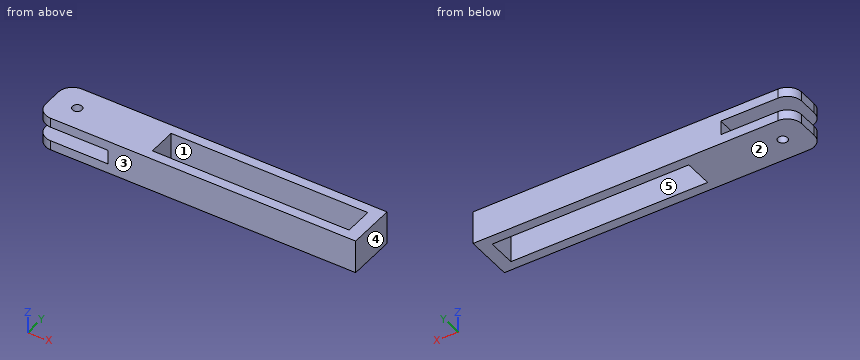
from build123d import *

# Parameters (mm, degrees)
SKETCH3_W           = 206.383928572
SKETCH3_H           = 30
BOSS_EXTRUDE1_DEPTH = 35
CUT_EXTRUDE2_REACH  = 180.273
SKETCH5_W           = 75
SKETCH5_H           = 15
SKETCH6_R           = 5
CUT_EXTRUDE3_DEPTH  = 173.934236055


with BuildPart() as part:
    # Sketch3 → Boss-Extrude1 (new body)
    with BuildSketch(Plane.XY):
        with BuildLine():
            Line((-167.5, 10), (-167.5, -10))
            ThreePointArc((-167.5, -10), (-163.106601718, -20.606601718), (-152.5, -25))
            Line((-152.5, -25), (167.5, -25))
            Line((167.5, -25), (167.5, 25))
            Line((167.5, 25), (-152.5, 25))
            ThreePointArc((-152.5, 25), (-163.106601718, 20.606601718), (-167.5, 10))
        make_face()
        with Locations((50.825520553, 0)):
            Rectangle(SKETCH3_W, SKETCH3_H, mode=Mode.SUBTRACT)
    extrude(amount=BOSS_EXTRUDE1_DEPTH)

    # Sketch5 → Cut-Extrude2 (cut, up to next)
    with BuildSketch(Plane.XZ.offset(25), mode=Mode.PRIVATE) as cut_extrude2_sk1:
        with Locations((-130, 17.5)):
            Rectangle(SKETCH5_W, SKETCH5_H)
    cut_extrude2_tool1 = extrude(cut_extrude2_sk1.sketch, amount=-CUT_EXTRUDE2_REACH, mode=Mode.PRIVATE) & part.part
    add(cut_extrude2_tool1.solids().sort_by_distance((-130, -25, 17.5))[0], mode=Mode.SUBTRACT)

    # Sketch6 → Cut-Extrude3 (cut, through all)
    with BuildSketch(Plane(origin=(0, 0, 0), x_dir=(-1, 0, 0), z_dir=(0, 0, -1))):
        with Locations((141.050190179, 0)):
            Circle(SKETCH6_R)
    extrude(amount=-CUT_EXTRUDE3_DEPTH, mode=Mode.SUBTRACT)


solid = part.part
Input: part model. Units: mm. Frame: model coordinates. Face numbers are marked on the shaded views. A direction names the side the tool comes from. Round coordinates to 2 decimals unless told otherwise and drop trailing zeros. Loops run counter-clockwise (first coordinate to the right, second up) from the corner with the lowest first, then second, coordinate; pieces in that order, holes last. Notation, with made-up numbers: (72.5, -40) -> (84.5, -40) arc R13 ccw to (84.5, -17) -> close; hole circle Ø9 at (25, -1.5). An arc over 180 degrees is marked (long way). Answer as a JSON object with one key per item and string values. Group by question number.
1) Section query C-C on x = 133.5. Output: boundary loops of the cut face in (y, z), plus the area to 3 significant figures.
2) Section query D-D on y = -22. Output: boundary loops of the cut face in (x, z).
3) Section query B-B on y = 0. Output: boundary loops of the cut face in (x, z), plus the area to 3 significant figures.
4) Draft query along X for the marked faces 3, 4 and 5. Return one class per face: +X half, -X half, draft (parallel to the pull), parting line (faces both ways), or undercut.
5) Section query A-A on z = 22. Output: boundary loops of the cut face in (x, y), plus the area to 3 significant figures.
6) Ray query, L1, parallel to Z at x = -145, y = -13; L2, parallel to X at y = -7.5, z = 13.5; L3, parallel to Y at x = 114, z = 4. Return the intervals inside material, ascending.
7) Reachability of the marked faces 1 and 2 from +Z, -Z, +X, -X, +Y, -Y: full face, straight path, thin tool, end or side. Return the list, or none.
8) Pin query (flat end, axial travel): pin 1 (1.5 mm diameter, centred on y = 1, z = 13, fed in from -X); pin 2 (9 mm diameter, centred on x = -141.05, y = 0, fed in from -Z). Return the tip coordinate at first contact, or that it passes through.
Reply:
{
 "1": {"outline": "(-25, 0) -> (-15, 0) -> (-15, 35) -> (-25, 35) -> close; (15, 0) -> (25, 0) -> (25, 35) -> (15, 35) -> close", "area": "700 mm2"},
 "2": {"outline": "(-161.5, 0) -> (167.5, 0) -> (167.5, 35) -> (-161.5, 35) -> (-161.5, 25) -> (-92.5, 25) -> (-92.5, 10) -> (-161.5, 10) -> close"},
 "3": {"outline": "(-167.5, 0) -> (-146.05, 0) -> (-146.05, 10) -> (-167.5, 10) -> close; (-167.5, 25) -> (-146.05, 25) -> (-146.05, 35) -> (-167.5, 35) -> close; (-136.05, 0) -> (-52.37, 0) -> (-52.37, 35) -> (-136.05, 35) -> (-136.05, 25) -> (-92.5, 25) -> (-92.5, 10) -> (-136.05, 10) -> close; (154.02, 0) -> (167.5, 0) -> (167.5, 35) -> (154.02, 35) -> close", "area": "3,180 mm2"},
 "4": {"face 3": "draft", "face 4": "+X half", "face 5": "undercut"},
 "5": {"outline": "(-92.5, -25) -> (167.5, -25) -> (167.5, 25) -> (-92.5, 25) -> close; hole (-52.37, -15) -> (154.02, -15) -> (154.02, 15) -> (-52.37, 15) -> close", "area": "6,810 mm2"},
 "6": {"L1": "z = 0 to 10, 25 to 35", "L2": "x = -92.5 to -52.37, 154.02 to 167.5", "L3": "y = -25 to -15, 15 to 25"},
 "7": {"face 1": "+Z, -Z", "face 2": "-Z, +X, -X, +Y, -Y"},
 "8": {"pin 1": "stops at x = -92.5", "pin 2": "passes through"}
}
